The drawing under review shows one solid part. Ordinate dimensions are in mm from its lowest x, y, z. Round coordinates to 2 decimals unless told otherwise and drop trailing zeros. Order: outer loops, then holes, each group sorted by start corner. A loop starts at its lowest first (then second) coordinate and runs counter-clockwise, first axis right, second up. Notation, with made-up numbers: M 21,-26.5 L 69,-26.5 A10 cw 69,-18.5 Z; hole C -22,71 d3. An arc over 180 degrees is marked long. Answer in a Markdown table with one row per item. Add a question column.
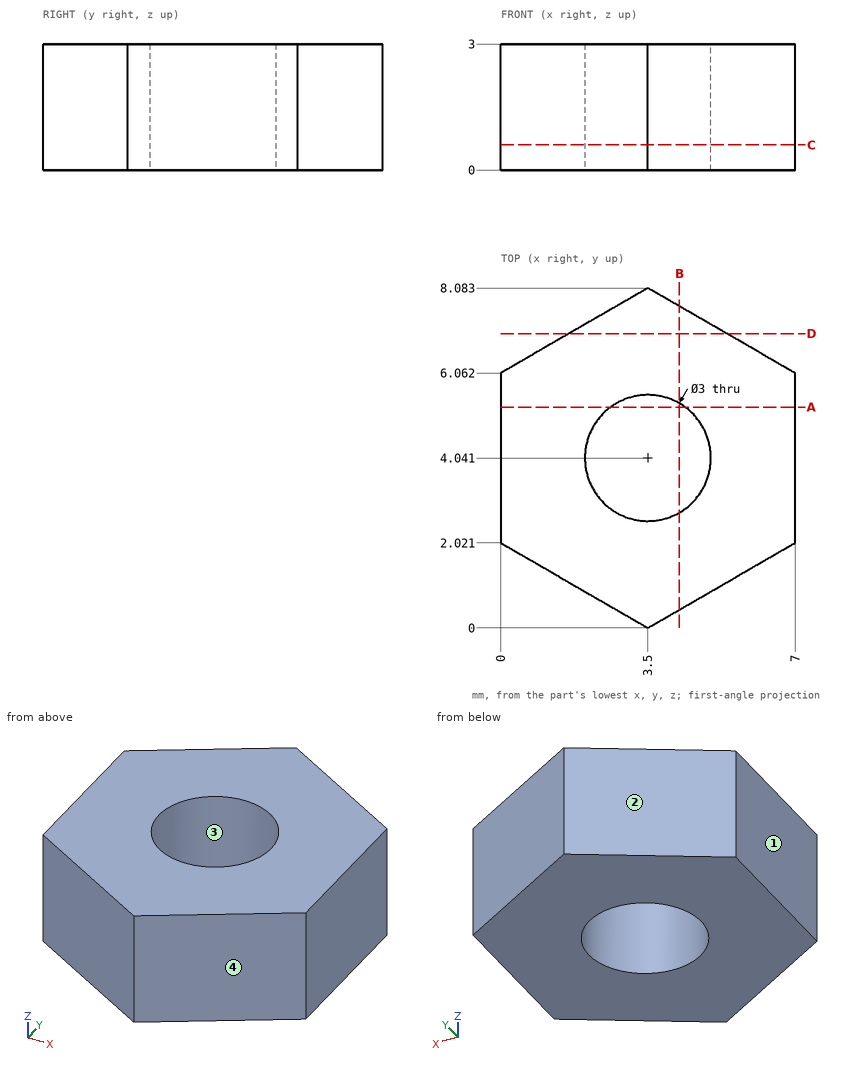
1. Consider section C-C on z = 0.6. Write out the cut boundary in (x, y).
2. Consider section B-B on x = 4.25. Write out the cut boundary in (y, z).
3. Consider section D-D on y = 7. Write out the cut boundary in (x, z) (1 decimal).
4. To check wall thickness, follow probe 1 along Y at (x, z) = (3, 0.95) (1 decimal); probe 2 along X at (y, z) = (3.25, 1.35) (1 decimal); probe 3 along X at (y, z) = (2.75, 2.8) (1 decimal). State the ranges of each line that lie inside material, in increasing order. Write a range as [from, to].
5. Consider section A-A on y = 5.25. Write out the cut boundary in (x, z).
6. The part is to be moulded in two halves that separate along Y. For the marked faces 1, 2, 3 and 4, say which applies: pulls with the +Y half, pulls with the -Y half, needs draft (parallel to the pull), parting line crosses it, or undercut.
Solved:
| question | item | result |
|---|---|---|
| 1 | outline | M 0,2.02 L 3.5,0 L 7,2.02 L 7,6.06 L 3.5,8.08 L 0,6.06 Z; hole C 3.5,4.04 d3 |
| 2 | outline | M 0.43,0 L 2.74,0 L 2.74,3 L 0.43,3 Z; M 5.34,0 L 7.65,0 L 7.65,3 L 5.34,3 Z |
| 3 | outline | M 1.6,0 L 5.4,0 L 5.4,3 L 1.6,3 Z |
| 4 | probe 1 | y = [0.3, 2.6], [5.5, 7.8] |
| 4 | probe 2 | x = [0, 2.2], [4.8, 7] |
| 4 | probe 3 | x = [0, 2.7], [4.3, 7] |
| 5 | outline | M 0,0 L 2.61,0 L 2.61,3 L 0,3 Z; M 4.39,0 L 7,0 L 7,3 L 4.39,3 Z |
| 6 | face 1 | needs draft |
| 6 | face 2 | pulls with the +Y half |
| 6 | face 3 | undercut |
| 6 | face 4 | pulls with the -Y half |
